from build123d import *

# Parameters (mm, degrees)
ESQUISSE1_R             = 1.75
BASE_EXTRUSION_DEPTH    = 1
BASE_EXTRUSION_TAPER    = 8
CONG_1_R                = 0.5
ESQUISSE2_R             = 1
BOSS_EXTRU_1_DEPTH      = 8
CHANFREIN1_SIZE         = 0.25
ENL_V_MAT_EXTRU_1_DEPTH = 0.5
CONG_2_R                = 0.25


with BuildPart() as part:
    # Esquisse1 → Base-Extrusion (new body)
    with BuildSketch(Plane.XY):
        Circle(ESQUISSE1_R)
    extrude(amount=BASE_EXTRUSION_DEPTH, taper=BASE_EXTRUSION_TAPER)

    # Congé1
    cong_1_edges = [part.edges().sort_by_distance(p)[0] for p in [
        (-1.609459165, 0, 1),
    ]]
    fillet(cong_1_edges, radius=CONG_1_R)

    # Esquisse2 → Boss.-Extru.1 (add)
    with BuildSketch(Plane(origin=(0, 0, 0), x_dir=(-1, 0, 0), z_dir=(0, 0, -1))):
        Circle(ESQUISSE2_R)
    extrude(amount=BOSS_EXTRU_1_DEPTH)

    # Chanfrein1
    chanfrein1_edges = [part.edges().sort_by_distance(p)[0] for p in [
        (1, 0, -8),
    ]]
    chamfer(chanfrein1_edges, length=CHANFREIN1_SIZE)

    # Esquisse3 → Enlèv. mat.-Extru.1 (cut)
    with BuildSketch(Plane.XY.offset(1)):
        Polygon((-0.125, 1), (-0.125, 0.125), (-1, 0.125), (-1, -0.125), (-0.125, -0.125), (-0.125, -1), (0.125, -1), (0.125, -0.125), (1, -0.125), (1, 0.125), (0.125, 0.125), (0.125, 1), align=None)
    extrude(amount=-ENL_V_MAT_EXTRU_1_DEPTH, mode=Mode.SUBTRACT)

    # Congé2
    cong_2_edges = [part.edges().sort_by_distance(p)[0] for p in [
        (-1.75, 0, 0),
    ]]
    fillet(cong_2_edges, radius=CONG_2_R)


solid = part.part
Can you work these out from the model? Positions are in its coordinate system, mm. A direction names the side the tool comes from. Coordinates: 2 decimals unless noted, no trailing zeros. Loops run counter-clockwise (first coordinate to the right, second up) from the corner with the lowest first, then second, coordinate; pieces in that order, holes last. Notation, with made-up numbers: M 36.5,82.25 L 88.5,82.25 A16 cw 88.5,110.25 Z; hole C 61,14.5 d11. An arc over 180 degrees is marked long. Answer as CSV lines item,"result". Start each with the question number.
1. Suppose I cut it at C-C, the plane z = -6.25. List the corners of the cut face in (x, y) for me, plus the area to 3 significant figures.
2. If I drill on probe 1 along Y at (x, z) = (-0.05, -7.5); probe 2 along Z at (x, y) = (-0.6, -0.95); probe 3 along Z at (x, y) = (0.05, -0.6), over which ranges is the centre line in solid material (lowest first)? Write a range as [from, to].
3. Thinking about a two-plate mould opening in X: for faces 3 (the face through (-0.3, 0.3, 1)), 4 (the face through (0, 0, 0.5)), 5 (the face through (0, -1, -4)), which applies, +X half, -X half, draft (parallel to the pull), parting line (faces both ways), or undercut?
4. For faces 1 (the face through (0.6, -1, 0)), 2 (the face through (0, 0, -8)), which set-ups out of +Z, -Z, +X, -X, +Y, -Y let a thin tool reach every point of the face, with its end or its side?
5. For pin 1 Ø0.6 at (x, z) = (-0.5, 0.5) entering from +Y; pin 2 Ø1 at (x, y) = (0.5, -1) entering from -Z, each with a flat end and sliding along its axis, tell me the tip position at first contact or that it passes through.
6. Suppose I cut it at A-A, the plane y = 0. List the corners of the cut face in (x, z) for me, plus the area to 3 significant figures.
Output:
1,outline,"C 0,0 d2"
1,area,"3.14 mm^2"
2,probe 1,"y = [-1, 1]"
2,probe 2,"z = [0, 1]"
2,probe 3,"z = [-8, 0.5]"
3,face 3,"draft"
3,face 4,"undercut"
3,face 5,"parting line"
4,face 1,"-Z"
4,face 2,"-Z, +X, -X, +Y, -Y"
5,pin 1,"stops at y = 1.69"
5,pin 2,"stops at z = -8"
6,outline,"M -1.71,0.28 A0.25 ccw -1.46,0 L -1,0 L -1,-7.75 L -0.75,-8 L 0.75,-8 L 1,-7.75 L 1,0 L 1.46,0 A0.25 ccw 1.71,0.28 L 1.67,0.57 A0.5 ccw 1.17,1 L 1,1 L 1,0.5 L -1,0.5 L -1,1 L -1.17,1 A0.5 ccw -1.67,0.57 Z"
6,area,"18.2 mm^2"
